The listing builds one solid part. Answer for the finished solid, in the listing's coordinates (mm). A direction names the side the tool comes from. Round coordinates to 2 decimals unless told otherwise and drop trailing zeros. Order: outer loops, then holes, each group sorted by start corner. A loop starts at its lowest first (then second) coordinate and runs counter-clockwise, first axis right, second up. Notation, with made-up numbers: M 67,71 L 82,71 A35 ccw 82,105 Z; hole C 34,-9.5 d7. An arc over 180 degrees is marked long. Put each result on its own line as item: value. Start each with the question number.
1. Consider line 1 (X direction, y = -1, z = 41); line 2 (Z direction, x = -23.5, y = 0); line 3 (Z direction, x = -16, y = 3). Determine where each line is inside the solid, lowest interval first.
2. The part is cut by section D-D (z = -40.5). Give the vertices of the cut face in (x, y), then the cut area to 3 significant figures.
3. The part is cut by section B-B (z = 58). Give the vertices of the cut face in (x, y), then the cut area to 3 significant figures.
4. The mould has two halves that part along Z. Classify faces 6 (the face through (-27.838, 0, -69)), 7 (the face through (0, 2, -67.45)), 8 (the face through (-29.68, -1.28, -66.68)), 9 (the face through (19.24, 2.28, 64.05)): +Z half, -Z half, draft (parallel to the pull), parting line (faces both ways), or undercut.
5. Which of the six approach directions +Z, -Z, +X, -X, +Y, -Y give full straight-line access (tool end or side, diameter ignored) to faces 1 (the face through (16.331, 2.282, 53.592)), 2 (the face through (-28.068, 2.826, 27.226)), 3 (the face through (-31.47, -0.05, -68.424)), 4 (the face through (-30.418, -1, 58)), 5 (the face through (-28, 2, 51.408))?
6. The part is cut by section A-A (x = -24.5). Give the vertices of the cut face in (y, z), then the cut area to 3 significant figures.
7. Each of these flat-tipped pins is pushed along its axis until it touches: pin 1 Ø2 at (y, z) = (-0.5, -69) entering from -X; pin 2 Ø2 at (x, y) = (3, 2) entering from -Z; pin 3 Ø3.5 at (x, y) = (-29.5, -0.5) entering from +Z; pin 4 Ø0.5 at (y, z) = (2, 35) entering from -X. Where does it stop, or does it pass through?
8. The part is cut by section C-C (x = -11). Give the vertices of the cut face in (y, z), then the cut area to 3 significant figures.
from build123d import *

# Parameters (mm, degrees)
F0_W      = 65.8367946744
F0_H      = 139.9032026529
F1_DEPTH  = 3.55
F2_R      = 5.08
F3_T      = -2.5
F5_DEPTH  = 12.7
F6_W      = 55.6767946744
F6_H      = 7.1
F7_DEPTH  = 2.5019
F8_W      = 7.1
F8_H      = 9.0527832508
F8_R      = 2.8313125725
F8_R_2    = 2.8285937047
F9_DEPTH  = 12.7
F10_DEPTH = 0.5


# Not quite as in the source:
# - a feature names something its author has since deleted; it is built from what else it names


with BuildPart() as f1:
    # F0 (on Front) → F1 (new body, symmetric)
    with BuildSketch(Plane.XZ):
        Rectangle(F0_W, F0_H)
    extrude(amount=F1_DEPTH, both=True)

    # F2
    f2_edges = [f1.edges().sort_by_distance(p)[0] for p in [
        (-32.918397, 0, 69.951601),
        (32.918397, 0, 69.951601),
        (-32.918397, 0, -69.951601),
        (32.918397, 0, -69.951601),
    ]]
    fillet(f2_edges, radius=F2_R)

    # F3
    f3_openings = [f1.faces().sort_by_distance(p)[0] for p in [
        (0, -3.55, 0),
    ]]
    offset(amount=F3_T, openings=f3_openings)

    # F4 (on Front) → F5 (cut, symmetric)
    with BuildSketch(Plane.XZ):
        Polygon((12.9001184621, 55.8146053817), (19.8599101564, 51.3060083088), (26.2985346927, 56.5319304354), (23.3180318028, 64.2703250051), (15.0373551768, 63.8269937409), align=None)
    extrude(amount=F5_DEPTH, both=True, mode=Mode.SUBTRACT)

    # F6 (on face) → F7 (cut, symmetric)
    with BuildSketch(Plane(origin=(0, 0, -69.9516013265), x_dir=(1, 0, 0), z_dir=(0, 0, -1))):
        Rectangle(F6_W, F6_H)
    extrude(amount=F7_DEPTH, both=True, mode=Mode.SUBTRACT)

    # F8 (on face) → F9 (cut, symmetric)
    with BuildSketch(Plane(origin=(-32.9183973372, 0, 0), x_dir=(0, -1, 0), z_dir=(-1, 0, 0))):
        with Locations((0, 46.8815155327)):
            Rectangle(F8_W, F8_H)
        with Locations((0, 34.2498570681)):
            Circle(F8_R)
        with Locations((0, 27.1013174206)):
            Circle(F8_R_2)
    extrude(amount=F9_DEPTH, both=True, mode=Mode.SUBTRACT)

    # F8 (on face) → F10 (cut, symmetric)
    with BuildSketch(Plane(origin=(-32.9183973372, 0, 0), x_dir=(0, -1, 0), z_dir=(-1, 0, 0))):
        with Locations((0, 46.8815155327)):
            Rectangle(F8_W, F8_H)
        with Locations((0, 34.2498570681)):
            Circle(F8_R)
        with Locations((0, 27.1013174206)):
            Circle(F8_R_2)
    extrude(amount=F10_DEPTH, both=True, mode=Mode.SUBTRACT)


solid = f1.part
Resolved:
1. line 1: -32.92 to -30.42, 30.42 to 32.92
1. line 2: 67.45 to 69.95
1. line 3: -67.45 to 69.95
2. outline: M -32.92,-3.55 L -30.42,-3.55 L -30.42,1.05 L 30.42,1.05 L 30.42,-3.55 L 32.92,-3.55 L 32.92,3.55 L -32.92,3.55 Z
2. area: 188 mm2
3. outline: M -32.92,-3.55 L -30.42,-3.55 L -30.42,1.05 L 13.48,1.05 L 13.48,3.55 L -32.92,3.55 Z; M 25.73,1.05 L 30.42,1.05 L 30.42,-3.55 L 32.92,-3.55 L 32.92,3.55 L 25.73,3.55 Z
3. area: 157 mm2
4. face 6: draft
4. face 7: -Z half
4. face 8: undercut
4. face 9: undercut
5. face 1: +Y, -Y
5. face 2: -X
5. face 3: -Z, -X, +Y, -Y
5. face 4: -Y
5. face 5: -X, +Y, -Y
6. outline: M -3.55,67.45 L 1.05,67.45 L 1.05,51.41 L 3.55,51.41 L 3.55,69.95 L -3.55,69.95 Z; M 1.05,-67.45 L 3.55,-67.45 L 3.55,42.36 L 1.05,42.36 L 1.05,36.88 A2.83 cw 1.05,31.62 L 1.05,29.73 A2.83 cw 1.05,24.47 Z
6. area: 319 mm2
7. pin 1: x = -31.84
7. pin 2: z = -67.45
7. pin 3: z = 69.95
7. pin 4: x = -20.22
8. outline: M -3.55,67.45 L 1.05,67.45 L 1.05,-67.45 L 3.55,-67.45 L 3.55,69.95 L -3.55,69.95 Z
8. area: 355 mm2
